from build123d import *

# Parameters (mm, degrees)
SKETCH1_R           = 3.5
SKETCH1_R_2         = 3.175
SKETCH1_R_3         = 1.778
BOSS_EXTRUDE1_DEPTH = 4.7625


with BuildPart() as part:
    # Sketch1 → Boss-Extrude1 (new body)
    with BuildSketch(Plane(origin=(0, 0, 0), x_dir=(1, 0, 0), z_dir=(0, 1, 0))):
        with BuildLine():
            Line((-82.138222173, -9.295950869), (-57.965959984, -9.295950869))
            ThreePointArc((-57.965959984, -9.295950869), (-55.705057174, -9.996205654), (-54.23575837, -11.851791627))
            ThreePointArc((-54.23575837, -11.851791627), (-25.688309848, -49.851999329), (18.508323348, -67.334282266))
            ThreePointArc((18.508323348, -67.334282266), (43.48483848, -72.142696572), (67.225777827, -81.270399198))
            ThreePointArc((67.225777827, -81.270399198), (68.831606216, -82.733374325), (69.400777827, -84.829805749))
            Line((69.400777827, -84.829805749), (69.400777827, -96.829805749))
            ThreePointArc((69.400777827, -96.829805749), (70.572350702, -99.658232874), (73.400777827, -100.829805749))
            Line((73.400777827, -100.829805749), (88.810777827, -100.829805749))
            ThreePointArc((88.810777827, -100.829805749), (91.639204952, -99.658232874), (92.810777827, -96.829805749))
            Line((92.810777827, -96.829805749), (92.810777827, -95.010813721))
            ThreePointArc((92.810777827, -95.010813721), (93.982350702, -92.182386597), (96.810777827, -91.010813721))
            Line((96.810777827, -91.010813721), (136.939777827, -91.010813721))
            Line((136.939777827, -91.010813721), (136.939777827, 48.804049131))
            Line((136.939777827, 48.804049131), (112.767515638, 48.804049131))
            ThreePointArc((112.767515638, 48.804049131), (110.506612828, 49.504303916), (109.037314024, 51.359889889))
            ThreePointArc((109.037314024, 51.359889889), (82.815823158, 87.522965038), (42.165907723, 106.041036281))
            ThreePointArc((42.165907723, 106.041036281), (13.766481711, 113.962861296), (-12.424222173, 127.502792592))
            ThreePointArc((-12.424222173, 127.502792592), (-14.009500528, 128.976393784), (-14.59507652, 131.060070509))
            Line((-14.59507652, 131.060070509), (-14.59507652, 157.379549131))
            ThreePointArc((-14.59507652, 157.379549131), (-15.766649396, 160.207976256), (-18.59507652, 161.379549131))
            Line((-18.59507652, 161.379549131), (-34.009222173, 161.379549131))
            ThreePointArc((-34.009222173, 161.379549131), (-36.837649298, 160.207976256), (-38.009222173, 157.379549131))
            Line((-38.009222173, 157.379549131), (-38.009222173, 134.518911983))
            ThreePointArc((-38.009222173, 134.518911983), (-39.180795048, 131.690484859), (-42.009222173, 130.518911983))
            Line((-42.009222173, 130.518911983), (-82.138222173, 130.518911983))
            Line((-82.138222173, 130.518911983), (-82.138222173, -9.295950869))
        make_face()
        with Locations((52.400777827, 44.754049131)):
            Circle(SKETCH1_R, mode=Mode.SUBTRACT)
        with Locations((52.400777827, -5.245950869)):
            Circle(SKETCH1_R, mode=Mode.SUBTRACT)
        with Locations((80.400777827, 9.550885679)):
            Circle(SKETCH1_R_2, mode=Mode.SUBTRACT)
        with Locations((109.880393645, 33.224433313)):
            Circle(SKETCH1_R_3, mode=Mode.SUBTRACT)
        with Locations((109.880393645, 6.283664949)):
            Circle(SKETCH1_R_3, mode=Mode.SUBTRACT)
        with Locations((109.880393645, -48.53042954)):
            Circle(SKETCH1_R_3, mode=Mode.SUBTRACT)
        with Locations((109.880393645, -75.471197903)):
            Circle(SKETCH1_R_3, mode=Mode.SUBTRACT)
        with Locations((130.26557504, -49.865610934)):
            Circle(SKETCH1_R_3, mode=Mode.SUBTRACT)
        with Locations((130.26557504, -74.136016508)):
            Circle(SKETCH1_R_3, mode=Mode.SUBTRACT)
        with Locations((130.26557504, 31.889251918)):
            Circle(SKETCH1_R_3, mode=Mode.SUBTRACT)
        with Locations((130.26557504, 7.618846344)):
            Circle(SKETCH1_R_3, mode=Mode.SUBTRACT)
        with Locations((80.400777827, -90.985264901)):
            Circle(SKETCH1_R_2, mode=Mode.SUBTRACT)
        with Locations((2.400777827, -5.245950869)):
            Circle(SKETCH1_R, mode=Mode.SUBTRACT)
        with Locations((2.400777827, 44.754049131)):
            Circle(SKETCH1_R, mode=Mode.SUBTRACT)
        with Locations((-25.599222173, 29.957212583)):
            Circle(SKETCH1_R_2, mode=Mode.SUBTRACT)
        with Locations((-55.078837991, 6.283664949)):
            Circle(SKETCH1_R_3, mode=Mode.SUBTRACT)
        with Locations((-55.078837991, 33.224433313)):
            Circle(SKETCH1_R_3, mode=Mode.SUBTRACT)
        with Locations((-55.078837991, 88.038527802)):
            Circle(SKETCH1_R_3, mode=Mode.SUBTRACT)
        with Locations((-55.078837991, 114.979296165)):
            Circle(SKETCH1_R_3, mode=Mode.SUBTRACT)
        with Locations((-75.464019386, 89.373709197)):
            Circle(SKETCH1_R_3, mode=Mode.SUBTRACT)
        with Locations((-75.464019386, 113.64411477)):
            Circle(SKETCH1_R_3, mode=Mode.SUBTRACT)
        with Locations((-75.464019386, 7.618846344)):
            Circle(SKETCH1_R_3, mode=Mode.SUBTRACT)
        with Locations((-75.464019386, 31.889251918)):
            Circle(SKETCH1_R_3, mode=Mode.SUBTRACT)
        with Locations((-25.599222173, 130.493363164)):
            Circle(SKETCH1_R_2, mode=Mode.SUBTRACT)
    extrude(amount=BOSS_EXTRUDE1_DEPTH)


solid = part.part
The listing builds one solid part. Answer for the finished solid, in the listing's coordinates (mm). Give positions to 0.01 mm unless a question says otherwise; leave off trailing zeros. Order: outer loops, then holes, each group sorted by start corner. A loop starts at its lowest first (then second) coordinate and runs counter-clockwise, first axis right, second up. Notation, with made-up numbers: (-27, 75.5) -> (25, 75.5) arc R17 cw to (25, 108.5) -> close; hole circle Ø9 at (28.5, 23). An arc over 180 degrees is marked (long way). Put each result on its own line as item: value.
Item 1: Given P1, Ø2.5, axis at x = 121.5, y = 2, coming from the +Z side; P2, Ø5.5, axis at x = 2.4, z = -44.75, coming from the +Y side; P3, Ø1.5, axis at x = -22.5, y = 1.5, coming from the +Z side, each flat-ended and moving along its own axis, determine where each tip first touches the part or whether it passes through.
Established:
P1: stops at z = 91.01
P2: passes through
P3: stops at z = 52.69
Item 2: A cutting plane is placed at C-C on z = 28. Give the vertices of the cut face in (x, y).
Established:
outline: (-45.97, 0) -> (136.94, 0) -> (136.94, 4.76) -> (-45.97, 4.76) -> close
Item 3: Straight lines are drawn through the part: line 1 (Z direction, x = 82, y = 3.3); line 2 (X direction, y = 4.05, z = -47); line 3 (Z direction, x = -62.5, y = 3.85). For each, find the intervals that lie inside material, in ascending order.
Established:
line 1: z = -88.18 to -12.29, -6.81 to 88.24, 93.73 to 100.83
line 2: x = -82.14 to -0.28, 5.09 to 49.72, 55.09 to 136.94
line 3: z = -130.52 to 9.3
Item 4: For a pull along Z with two mould halves and no side action, classify faces 1 (the face through (49.623, 2.348, -42.624)), 2 (the face through (26, 0, -32)), 3 (the face through (49.623, 2.348, 7.376)), 4 (the face through (43.142, 2.348, 72.045)) as released by +Z, released by -Z, zero draft, split by the parting line, or undercut.
Established:
face 1: undercut
face 2: zero draft
face 3: undercut
face 4: released by +Z
Item 5: A cutting plane is placed at B-B on y = 1.9. Count the separate pieces of the cut face and the enclosed holes in it, plus the area to 3 significant figures.
Established:
separate pieces: 1
enclosed holes: 24
area: 37,000 mm^2
Item 6: A cutting plane is placed at A-A on x = -61. Give the vertices of the cut face in (y, z), plus the area to 3 significant figures.
Established:
outline: (0, -130.52) -> (4.76, -130.52) -> (4.76, 9.3) -> (0, 9.3) -> close
area: 666 mm^2
